Source: three-view drawing plus pictorial views. Frame: mm from the lowest corner of the part. A direction names the side the tool comes from. Round coordinates to 2 decimals unless told otherwise and drop trailing zeros. Order: outer loops, then holes, each group sorted by start corner. A loop starts at its lowest first (then second) coordinate and runs counter-clockwise, first axis right, second up. Notation, with made-up numbers: (-33, 52) - (-26, 52) arc R23 ccw to (-26, 91) - close; hole circle Ø9 at (14, 18.25). An arc over 180 degrees is marked (long way). Use one line per item in the form item = value. Start each with the question number.
Q1. Cut plane B-B, the plane y = 7.5. Return the cut outline in (x, z) (3 decimals).
Q2. Pin query (flat end, axial travel): pin 1 Ø5.5 at (x, y) = (12, 7.5) entering from -Z. Return the tip coordinate at first contact, or that it passes through.
Q3. Ray query, line 1 (Y direction, x = 10, z = 0.75) (3 decimals); line 2 (X direction, y = 5.25, z = 5) (3 decimals); line 3 (Z direction, x = 4.75, y = 8.5). Return the intervals inside material, ascending. Write a range as [from, to].
Q4. Cut plane A-A, the plane z = 6.75. Return the cut outline in (x, y) (3 decimals).
Q5. Set-up query: the marked faces 1 and 2. Return all of +Z, -Z, +X, -X, +Y, -Y with unobstructed straight access to the full face (end or side cutting, diameter ignored); none if empty.
Q6. Draft query along X for the marked faces 3, 4 and 5. Return one class per face: released by +X, released by -X, zero draft, split by the parting line, or undercut.
Q7. Cut plane C-C, the plane x = 9. Return the cut outline in (y, z) (3 decimals), and give its area (3 significant figures).
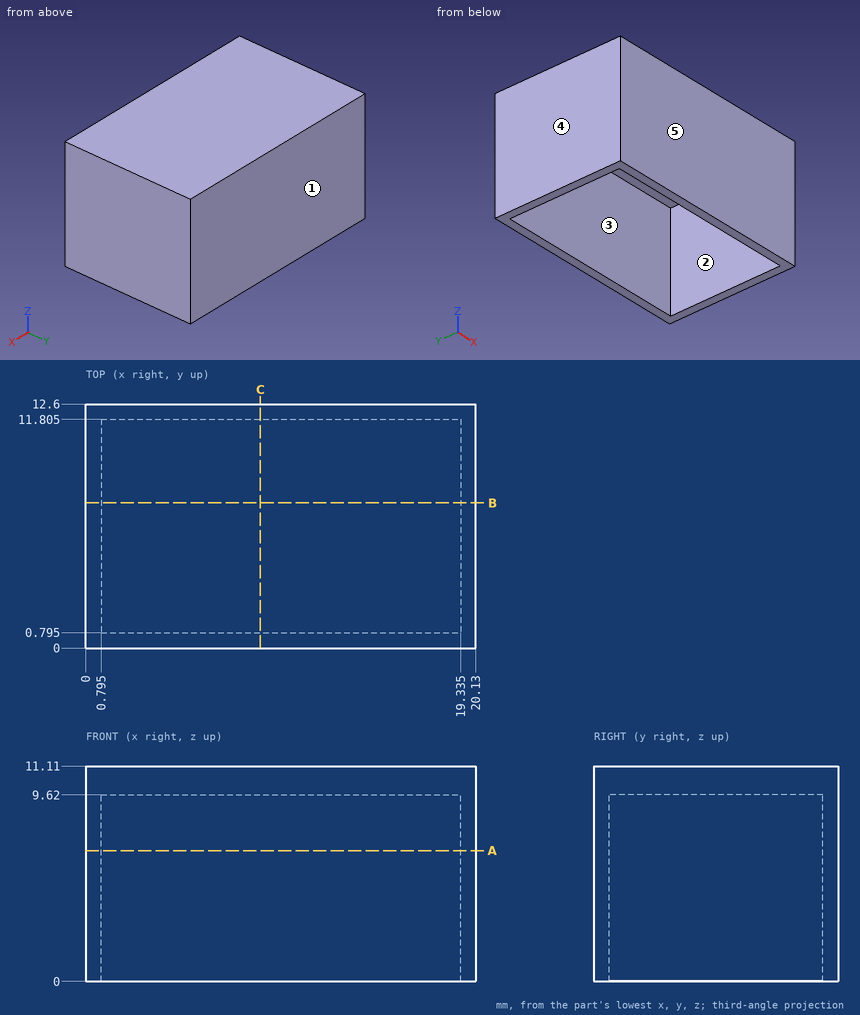
Completed:
q1.outline = (0, 0) - (0.795, 0) - (0.795, 9.62) - (19.335, 9.62) - (19.335, 0) - (20.13, 0) - (20.13, 11.11) - (0, 11.11) - close
q2.pin_1 = 9.62
q3.line_1 = [0, 0.795], [11.805, 12.6]
q3.line_2 = [0, 0.795], [19.335, 20.13]
q3.line_3 = [9.62, 11.11]
q4.outline = (0, 0) - (20.13, 0) - (20.13, 12.6) - (0, 12.6) - close; hole (0.795, 0.795) - (19.335, 0.795) - (19.335, 11.805) - (0.795, 11.805) - close
q5.face_1 = +Z, -Z, +X, -X, +Y
q5.face_2 = -Z
q6.face_3 = undercut
q6.face_4 = released by -X
q6.face_5 = zero draft
q7.outline = (0, 0) - (0.795, 0) - (0.795, 9.62) - (11.805, 9.62) - (11.805, 0) - (12.6, 0) - (12.6, 11.11) - (0, 11.11) - close
q7.area = 34.1 mm2
